Geometry check sheet. Reference: the model listing, model coordinates, mm. A direction names the side the tool comes from. Give positions to 0.01 mm unless a question says otherwise; leave off trailing zeros. Write each loop counter-clockwise with the first axis right and the second up, starting at its lowest first coordinate (ties: lowest second). Pieces come first, ordered by that corner, then holes. Notation, with made-up numbers: (3.5, 50.5) -> (51.5, 50.5) arc R20 ccw to (51.5, 66.5) -> close; hole circle Ø10 at (70.25, 46). An arc over 180 degrees is marked (long way). One line per item, written item: value.
from build123d import *

# Parameters (mm, degrees)
SKETCH1_W                      = 41
SKETCH1_H                      = 20
EXTRUDE1_DEPTH                 = 38
SKETCH2_W                      = 2.5
SKETCH2_H                      = 52
EXTRUDE2_DEPTH                 = 20
SKETCH3_R                      = 6.5
EXTRUDE3_DEPTH                 = 3.8
SKETCH4_R                      = 2.95
EXTRUDE4_DEPTH                 = 4.2
F_4_4_4_4_DIAMETER_HOLE1_D     = 4.4
F_4_4_4_4_DIAMETER_HOLE1_DEPTH = 150
F_4_4_4_4_DIAMETER_HOLE1_TIP   = 1.321893362


with BuildPart() as part:
    # Sketch1 → Extrude1 (new body)
    with BuildSketch(Plane.XY):
        with Locations((0.479801018, -0.224419429)):
            Rectangle(SKETCH1_W, SKETCH1_H)
    extrude(amount=EXTRUDE1_DEPTH)

    # Sketch2 → Extrude2 (add)
    with BuildSketch(Plane(origin=(0, 9.775580571, 0), x_dir=(1, 0, 0), z_dir=(0, 1, 0))):
        with Locations((-7.270198982, -19)):
            Rectangle(SKETCH2_W, SKETCH2_H)
    extrude(amount=-EXTRUDE2_DEPTH)

    # Sketch3 → Extrude3 (add)
    with BuildSketch(Plane.ZY.offset(20.020198982)):
        with Locations((28.3, 0)):
            Circle(SKETCH3_R)
    extrude(amount=EXTRUDE3_DEPTH)

    # Sketch4 → Extrude4 (add)
    with BuildSketch(Plane.ZY.offset(23.820198982)):
        with Locations((28.3, 0)):
            Circle(SKETCH4_R)
    extrude(amount=EXTRUDE4_DEPTH)

    # Ø4.4 (4.4) Diameter Hole1
    with Locations(Plane(origin=(-8.520198982, 4.860580571, -4.63), x_dir=(0, 0, -1), z_dir=(-1, 0, 0))):
        with Locations((0, 0), (0, 10.17), (-47.26, 0), (-47.26, 10.17)):
            Hole(F_4_4_4_4_DIAMETER_HOLE1_D / 2, depth=F_4_4_4_4_DIAMETER_HOLE1_DEPTH)
            with Locations((0, 0, -(F_4_4_4_4_DIAMETER_HOLE1_DEPTH + F_4_4_4_4_DIAMETER_HOLE1_TIP / 2))):  # 118° drill point
                Cone(0, F_4_4_4_4_DIAMETER_HOLE1_D / 2, F_4_4_4_4_DIAMETER_HOLE1_TIP, mode=Mode.SUBTRACT)


solid = part.part
1) Sectioned sample at D-D on z = 28.3. Record the cut outline in (x, y).
Verdict:
outline: (-28.02, -2.95) -> (-23.82, -2.95) -> (-23.82, -6.5) -> (-20.02, -6.5) -> (-20.02, -10.22) -> (20.98, -10.22) -> (20.98, 9.78) -> (-20.02, 9.78) -> (-20.02, 6.5) -> (-23.82, 6.5) -> (-23.82, 2.95) -> (-28.02, 2.95) -> close
2) Sectioned sample at C-C on y = 0. Record the cut outline in (x, z).
Verdict:
outline: (-28.02, 25.35) -> (-23.82, 25.35) -> (-23.82, 21.8) -> (-20.02, 21.8) -> (-20.02, 0) -> (-8.52, 0) -> (-8.52, -7) -> (-6.02, -7) -> (-6.02, 0) -> (20.98, 0) -> (20.98, 38) -> (-6.02, 38) -> (-6.02, 45) -> (-8.52, 45) -> (-8.52, 38) -> (-20.02, 38) -> (-20.02, 34.8) -> (-23.82, 34.8) -> (-23.82, 31.25) -> (-28.02, 31.25) -> close
3) Depth check by flat-ended pin: pin 1 Ø1.5 at (x, y) = (3.5, 5.5) entering from -Z; pin 2 Ø3.5 at (y, z) = (-3, 42.5) entering from -X; pin 3 Ø4 at (x, y) = (0, -3) entering from +Z. Enter the tip coordinate at first touch or a pass-through.
Verdict:
pin 1: z = 0
pin 2: x = -8.52
pin 3: z = 38
4) Tool access check on faces 4 (the cylindrical face through (-21.9, -2.5, 34.3)), 5 (the flat face through (-14, 0, 38)), 6 (the flat face through (7, 0, 0)), 7 (the flat face through (-14, 0, 0)), 8 (the flat face through (-6.02, 0, 42)). Record the directions out of +Z, -Z, +X, -X, +Y, -Y that give a thin tool (end or side, any length) a straight path to the whole face; none if there is none.
Verdict:
face 4: -X
face 5: +Z, -X, +Y, -Y
face 6: -Z, +X, +Y, -Y
face 7: -Z, -X, +Y, -Y
face 8: +Z, +X, +Y, -Y
5) Mould release check, pull along X, two halves, no side actions. Record for faces 1 (the flat face through (-8.52, 0, 42)), 2 (the flat face through (-6.02, 0, -3)), 3 (the flat face through (0, -10.224, 19)): released by +X, released by -X, zero draft, split by the parting line, or undercut.
Verdict:
face 1: released by -X
face 2: released by +X
face 3: zero draft
6) Scan lines: probe 1 along Y at (x, z) = (-7.95, -4.63); probe 2 along Y at (x, z) = (-7, 42); probe 3 along Z at (x, y) = (15, 6.75). Record each from-to range of solid material in increasing order.
Verdict:
probe 1: -10.22 to -7.51, -3.11 to 2.66, 7.06 to 9.78
probe 2: -10.22 to -7.42, -3.2 to 2.75, 6.97 to 9.78
probe 3: 0 to 38
7) Sectioned sample at A-A on z = -4.63. Record the cut outline in (x, y).
Verdict:
outline: (-8.52, -10.22) -> (-6.02, -10.22) -> (-6.02, -7.51) -> (-8.52, -7.51) -> close; (-8.52, -3.11) -> (-6.02, -3.11) -> (-6.02, 2.66) -> (-8.52, 2.66) -> close; (-8.52, 7.06) -> (-6.02, 7.06) -> (-6.02, 9.78) -> (-8.52, 9.78) -> close
8) Sectioned sample at B-B on y = 4. Record the cut outline in (x, z), plus the area to 3 significant figures.
Verdict:
outline: (-23.82, 23.18) -> (-20.02, 23.18) -> (-20.02, 0) -> (-8.52, 0) -> (-8.52, -2.61) -> (-6.02, -2.61) -> (-6.02, 0) -> (20.98, 0) -> (20.98, 38) -> (-6.02, 38) -> (-6.02, 40.61) -> (-8.52, 40.61) -> (-8.52, 38) -> (-20.02, 38) -> (-20.02, 33.42) -> (-23.82, 33.42) -> close; (-8.52, -7) -> (-6.02, -7) -> (-6.02, -6.65) -> (-8.52, -6.65) -> close; (-8.52, 44.65) -> (-6.02, 44.65) -> (-6.02, 45) -> (-8.52, 45) -> close
area: 1,610 mm^2
